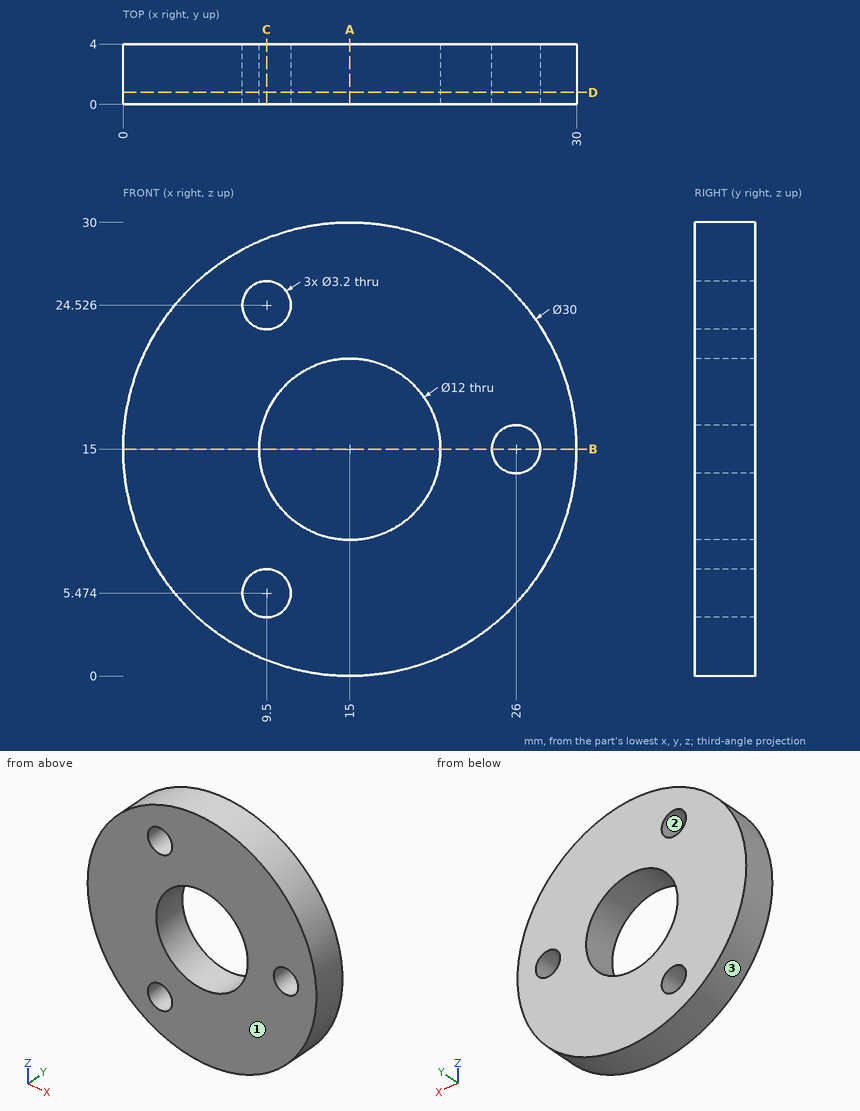
Answer from the drawing. Dimensions are ordinates in mm from the lowest x, y and z of the part. Give positions to 0.01 mm unless a question says otherwise; leave off trailing zeros. Loops run counter-clockwise (first coordinate to the right, second up) from the corner with the lowest first, then second, coordinate; pieces in that order, holes last.
Item 1: Find the intervals of material crossed by line 1 along X through (y, z) = (2.95, 15); line 2 along Z through (x, y) = (15, 1.45); line 3 along X through (y, z) = (2.6, 4.5), in increasing order.
Item 2: The part is cut by section B-B (z = 15). Write down the section's boundary in (x, y), and give its area (3 significant figures).
Item 3: The part is cut by section C-C (x = 9.5). Write down the section's boundary in (y, z) (1 decimal).
Item 4: The part is cut by section D-D (y = 0.8). Write down the section's boundary in (x, z).
Item 5: The mould has two halves that part along X. Classify the marked faces 1, 2 and 3: released by +X, released by -X, zero draft, split by the parting line, or undercut.
Item 6: The part is cut by section A-A (x = 15). Write down the section's boundary in (y, z).
Item 7: This flat-tipped pin is pushed along its axis until it touches: pin 1 Ø3.5 at (x, z) = (9.5, 5.47) entering from -Y. Where does it stop, or does it pass through?
Taken from the geometry:
1. line 1: x = 0 to 9, 21 to 24.4, 27.6 to 30
1. line 2: z = 0 to 9, 21 to 30
1. line 3: x = 4.29 to 8.23, 10.77 to 25.71
2. outline: (0, 0) - (9, 0) - (9, 4) - (0, 4) - close; (21, 0) - (24.4, 0) - (24.4, 4) - (21, 4) - close; (27.6, 0) - (30, 0) - (30, 4) - (27.6, 4) - close
2. area: 59.2 mm2
3. outline: (0, 1) - (4, 1) - (4, 3.9) - (0, 3.9) - close; (0, 7.1) - (4, 7.1) - (4, 12.6) - (0, 12.6) - close; (0, 17.4) - (4, 17.4) - (4, 22.9) - (0, 22.9) - close; (0, 26.1) - (4, 26.1) - (4, 29) - (0, 29) - close
4. outline: circle Ø30 at (15, 15); hole circle Ø3.2 at (9.5, 5.47); hole circle Ø3.2 at (9.5, 24.53); hole circle Ø12 at (15, 15); hole circle Ø3.2 at (26, 15)
5. face 1: zero draft
5. face 2: undercut
5. face 3: split by the parting line
6. outline: (0, 0) - (4, 0) - (4, 9) - (0, 9) - close; (0, 21) - (4, 21) - (4, 30) - (0, 30) - close
7. pin 1: stops at y = 0
